Answer from the drawing. Dimensions are ordinates in mm from the lowest x, y and z of the part. A direction names the side the tool comes from. Coordinates: 2 decimals unless noted, no trailing zeros. Order: outer loops, then holes, each group sorted by start corner. A loop starts at its lowest first (then second) coordinate and runs counter-clockwise, first axis right, second up.
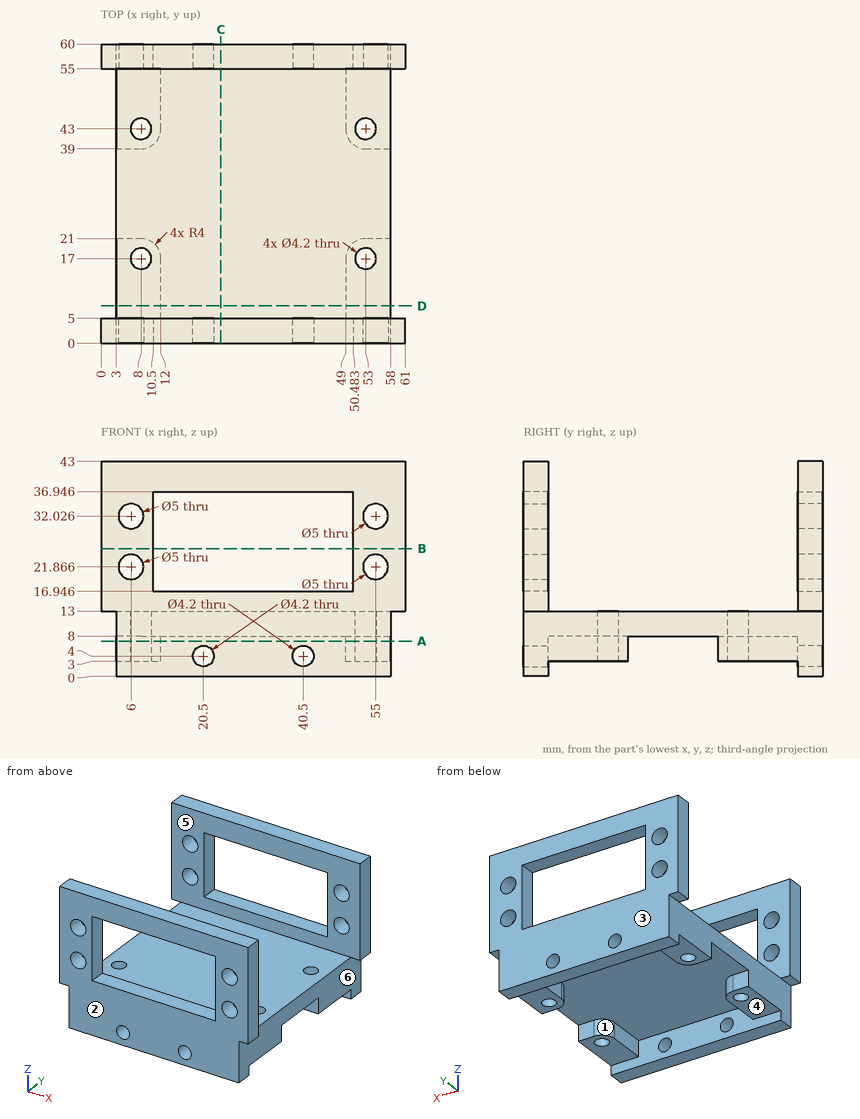
1) Determine the mould class of the marked faces 1, 2 and 3 for opening direction Y: released by +Y, released by -Y, zero draft, split by the parting line, or undercut.
2) Section A-A (z = 7) is taken. Give the vertices of the cut face in (x, y).
3) A tool of negligible diameter and unlimited length cuts with its end or side. For the marked faces 4, 5 and 6, from which of +Z, -Z, +X, -X, +Y, -Y can it reach the whole face along a straight path? Write none if from no direction.
4) Section C-C (x = 24) is taken. Give the vertices of the cut face in (y, z), then the cut area to 3 significant figures.
5) Each of these flat-tipped pins is pushed along its axis until it touches: P1, Ø6, axis at x = 32.5, y = 29, coming from the -Z side; P2, Ø12, axis at y = 13, z = 5, coming from the -X side; P3, Ø6.5, axis at x = 8, y = 43, coming from the +Z side. Where does it stop, or does it pass through?
6) Section D-D (y = 7.5) is taken. Give the vertices of the cut face in (x, z).
7) Consider L1, parallel to Y at x = 53, z = 10; L2, parallel to Y at x = 53, z = 6.5; L3, parallel to Z at x = 40.5, y = 57.35. Determine where each line is inside the solid, lowest interval first.
8) Section B-B (z = 25.5) is taken. Give the vertices of the cut face in (x, y), then the cut area to 3 significant figures.
Filled sheet:
1. face 1: undercut
1. face 2: released by -Y
1. face 3: released by +Y
2. outline: (3, 0) - (58, 0) - (58, 21) - (53, 21) arc R4 ccw to (49, 17) - (49, 5) - (12, 5) - (12, 17) arc R4 ccw to (8, 21) - (3, 21) - close; (3, 39) - (8, 39) arc R4 ccw to (12, 43) - (12, 55) - (49, 55) - (49, 43) arc R4 ccw to (53, 39) - (58, 39) - (58, 60) - (3, 60) - close; hole circle Ø4.2 at (8, 17); hole circle Ø4.2 at (8, 43); hole circle Ø4.2 at (53, 17); hole circle Ø4.2 at (53, 43)
3. face 4: -Z, +X, -X
3. face 5: +Z, +X, -X
3. face 6: -Z, +X, +Y, -Y
4. outline: (0, 0) - (5, 0) - (5, 8) - (55, 8) - (55, 0) - (60, 0) - (60, 16.95) - (55, 16.95) - (55, 13) - (5, 13) - (5, 16.95) - (0, 16.95) - close; (0, 36.95) - (5, 36.95) - (5, 43) - (0, 43) - close; (55, 36.95) - (60, 36.95) - (60, 43) - (55, 43) - close
4. area: 480 mm2
5. P1: stops at z = 8
5. P2: stops at x = 3
5. P3: stops at z = 13
6. outline: (3, 3) - (12, 3) - (12, 8) - (49, 8) - (49, 3) - (58, 3) - (58, 13) - (3, 13) - close
7. L1: y = 0 to 14.9, 19.1 to 40.9, 45.1 to 60
7. L2: y = 0 to 14.9, 19.1 to 21, 39 to 40.9, 45.1 to 60
7. L3: z = 0 to 1.9, 6.1 to 16.95, 36.95 to 43
8. outline: (0, 0) - (10.5, 0) - (10.5, 5) - (0, 5) - close; (0, 55) - (10.5, 55) - (10.5, 60) - (0, 60) - close; (50.48, 0) - (61, 0) - (61, 5) - (50.48, 5) - close; (50.48, 55) - (61, 55) - (61, 60) - (50.48, 60) - close
8. area: 210 mm2
